```python
from build123d import *

# Parameters (mm, degrees)
F0_R     = 9
F1_DEPTH = 3
F2_R     = 5
F3_DEPTH = 4.9
F4_R     = 4
F5_DEPTH = 15


with BuildPart() as f1:
    # F0 (on Top) → F1 (new body)
    with BuildSketch(Plane.XY):
        Circle(F0_R)
    extrude(amount=-F1_DEPTH)

    # F2 (on Top) → F3 (join)
    with BuildSketch(Plane.XY):
        Circle(F2_R)
    extrude(amount=F3_DEPTH)

    # F4 (on Top) → F5 (cut, symmetric)
    with BuildSketch(Plane.XY):
        Circle(F4_R)
    extrude(amount=F5_DEPTH, both=True, mode=Mode.SUBTRACT)


solid = f1.part
```
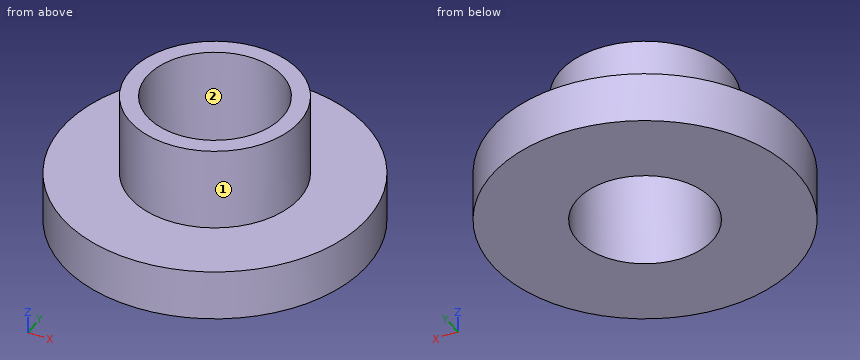
Read the model definition and answer for the solid it produces. Units are mm, in the model's axes. Face numbers are marked on the shaded views. A direction names the side the tool comes from. Coordinates: 2 decimals unless noted, no trailing zeros. Loops run counter-clockwise (first coordinate to the right, second up) from the corner with the lowest first, then second, coordinate; pieces in that order, holes last.
(1) Flat-ended cylindrical pins translate along their axes: pin 1 Ø4 at (x, y) = (-5.5, 7) entering from +Z; pin 2 Ø2 at (x, z) = (-4.5, 2.5) entering from -Y; pin 3 Ø4 at (y, z) = (4.5, 0) entering from -X. Find the tip coordinate at first contact, or state that the pin passes through.
Solution:
pin 1: stops at z = 0
pin 2: stops at y = -3.57
pin 3: stops at x = -8.65
(2) Consider line 1 along Y through (x, z) = (0, 3); line 2 along Z through (x, y) = (-2.25, -7.5); line 3 along X through (y, z) = (-3.25, -0.25). Determine where each line is inside the solid, lowest interval first.
Solution:
line 1: y = -5 to -4, 4 to 5
line 2: z = -3 to 0
line 3: x = -8.39 to -2.33, 2.33 to 8.39
(3) The part is cut by section A-A (y = 0). Determine the outline of the cut face in (x, z), and give its area (3 significant figures).
Solution:
outline: (-9, -3) - (-4, -3) - (-4, 4.9) - (-5, 4.9) - (-5, 0) - (-9, 0) - close; (4, -3) - (9, -3) - (9, 0) - (5, 0) - (5, 4.9) - (4, 4.9) - close
area: 39.8 mm2
(4) A tool of negligible diameter and unlimited length cuts with its end or side. For the marked faces 1 and 2, from which of +Z, -Z, +X, -X, +Y, -Y can it reach the whole face along a straight path? Write none if from no direction.
Solution:
face 1: +Z
face 2: +Z, -Z
(5) The part is cut by section D-D (x = 6). Determine the outline of the cut face in (y, z).
Solution:
outline: (-6.71, -3) - (6.71, -3) - (6.71, 0) - (-6.71, 0) - close
(6) The part is cut by section C-C (z = 4.5). Determine the outline of the cut face in (x, y), and give its area (3 significant figures).
Solution:
outline: circle Ø10 at (0, 0); hole circle Ø8 at (0, 0)
area: 28.3 mm2
